Input: part model. Units: mm. Frame: model coordinates. Round coordinates to 2 decimals unless told otherwise and drop trailing zeros. Order: outer loops, then holes, each group sorted by start corner. A loop starts at its lowest first (then second) coordinate and runs counter-clockwise, first axis right, second up. Notation, with made-up numbers: (-13, 12) -> (35, 12) arc R20 cw to (35, 43) -> close; hole circle Ø11 at (43.5, 20.25). An arc over 180 degrees is marked (long way). Answer as CSV lines item,"result". Start each with the question number.
1) Section query D-D, the plane z = 19. Output: boundary loops of the cut face in (x, y) (3 decimals).
2) Line query: L1, parallel to Z at x = -3.4, y = 142.24; L2, parallel to Z at x = -5.5, y = 130 (3 decimals); L3, parallel to X at y = 31, z = 76. Output: solid intervals per line, ascending.
3) Section query C-C, the plane y = 78. Output: boundary loops of the cut face in (x, z) (3 decimals), and give its area (3 significant figures).
4) Section query A-A, the plane z = 78.5. Output: boundary loops of the cut face in (x, y).
5) First-contact query: P1, Ø7.5, axis at y = 24.18, z = -24.05, coming from the -X side; P2, Ø3, axis at x = -9, y = 117.5, coming from the -Z side; P3, Ø10, axis at x = -18.5, y = -3, coming from the +Z side (3 decimals); P4, Ø4, axis at y = 19.5, z = -23, coming from the +X side. Flat tips, straight axial feed; report the tip coordinate or a pass-through.
6) Section query B-B, the plane x = -28. Output: boundary loops of the cut face in (y, z) (3 decimals), and give its area (3 significant figures).
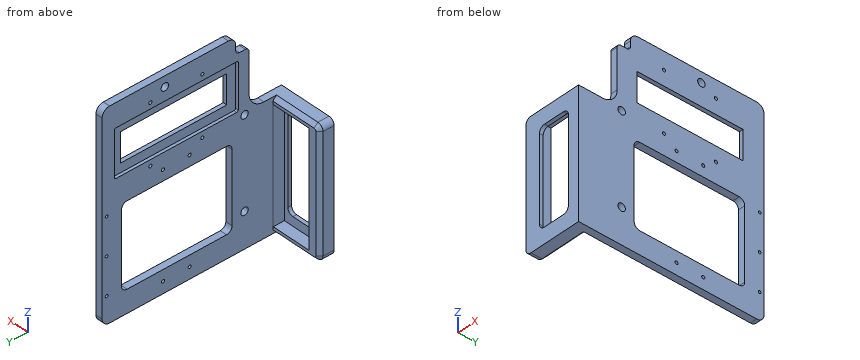
Autodesk Inventor part; units mm, degrees
ref_plane "YZ Plane" through (0, 0, 0) normal (1, 0, 0) x (0, 1, 0)
ref_plane "XZ Plane" through (0, 0, 0) normal (0, 1, 0) x (-1, 0, 0)
ref_plane "XY Plane" through (0, 0, 0) normal (0, 0, 1) x (1, 0, 0)
sketch "Sketch1" plane through (0, 0, 0) normal (0, 1, 0) x (-1, 0, 0)
  line L0 (0, -75.565) -> (0, 75.565)
  line L1 (-9.8806, 0) -> (59.2836, 0)
  line L2 (36.703, -40.64) -> (9.525, -40.64)
  line L3 (9.525, -40.64) -> (9.525, 40.64)
  line L4 (9.525, 40.64) -> (36.703, 40.64)
  line L5 (36.703, 40.64) -> (36.703, -40.64)
  line L6 (36.703, -40.64) -> (9.525, 40.64) construction
  line L7 (9.525, -40.64) -> (36.703, 40.64) construction
  line L8 (0, -53.975) -> (49.403, -53.975)
  line L9 (49.403, -53.975) -> (49.403, 53.975)
  line L10 (49.403, 53.975) -> (0, 53.975)
  line L11 (0, 53.975) -> (0, -53.975)
  line L12 (0, -53.975) -> (49.403, 53.975) construction
  line L13 (49.403, -53.975) -> (0, 53.975) construction
  point P0 (0, 0)
  point P1 (23.114, 0)
  point P2 (24.7015, 0)
  dimension "d0" = 81.28
  dimension "d1" = 27.178
  dimension "d3" = 107.95
  dimension "d4" = 12.7
  dimension "d6" = 9.525
  dimension "d7" = 0
extrude "Extrusion1" add sketch "Sketch1" against normal blind 12.7 contours L0 L1 L3 L2 L5 L9 L8 | L0 L10 L9 L1 L5 L4 L3
sketch "Sketch2" plane through (0, 0, 0) normal (0, 1, 0) x (1, 0, 0)
  point P0 (0, 0)
sketch "Sketch4" plane through (0, 0, 0) normal (0, 1, 0) x (1, 0, 0)
  point P0 (0, 0)
sketch "Sketch5" plane through (0, 0, 0) normal (0, 1, 0) x (1, 0, 0)
  line L0 (9.8806, 0) -> (-59.2836, 0)
  line L1 (0, 75.565) -> (0, -75.565)
  line L2 (-39.878, 48.26) -> (-6.223, 48.26)
  line L3 (-6.223, 48.26) -> (-6.223, -48.26)
  line L4 (-6.223, -48.26) -> (-39.878, -48.26)
  line L5 (-39.878, -48.26) -> (-39.878, 48.26)
  line L6 (-39.878, 48.26) -> (-6.223, -48.26) construction
  line L7 (-6.223, 48.26) -> (-39.878, -48.26) construction
  line L8 (-9.525, 40.64) -> (-9.525, -40.64)
  point P0 (0, 0)
  point P1 (-23.0505, 0)
  dimension "d13" = 3.302
  dimension "d14" = 96.52
  dimension "d15" = 33.655
extrude "Extrusion3" cut sketch "Sketch5" against normal blind 9.525
sketch "Sketch3" plane through (0, 0, 53.975) normal (1, 0, 0) x (0, 0, -1)
  line L0 (0, 0) -> (0, -12.7)
  line L1 (0, 0) -> (107.95, 0)
  line L2 (107.95, 0) -> (107.95, -12.7)
  line L3 (107.95, 146.05) -> (0, 146.05)
  line L4 (0, 146.05) -> (0, 0)
  line L5 (0, 0) -> (107.95, 0)
  line L6 (107.95, 0) -> (107.95, 146.05)
  line L7 (107.95, 146.05) -> (0, 0) construction
  line L8 (0, 146.05) -> (107.95, 0) construction
  line L9 (0, 20.32) -> (-63.5, 20.32)
  line L10 (-63.5, 20.32) -> (-63.5, 146.05)
  line L11 (-63.5, 146.05) -> (0, 146.05)
  line L12 (107.95, -12.7) -> (0, -12.7)
  line L13 (-49.53, 20.32) -> (-49.53, 31.75)
  line L14 (-49.53, 31.75) -> (-63.5, 31.75)
  point P0 (53.975, 0)
  point P1 (53.975, 73.025)
  point P2 (1.8288, 24.1808)
  point P3 (78.0288, 24.1808)
  point P4 (-54.7116, 92.3798)
  dimension "d10" = 146.05
  dimension "d18" = 33.02
  dimension "d19" = 63.5
  dimension "d20" = 13.97
  dimension "d21" = 11.43
  dimension "d22" = 36.8808
  dimension "d23" = 29.9212
  dimension "d24" = 106.1212
  dimension "d32" = 162.6616
  dimension "d33" = 105.0798
extrude "Extrusion2" add sketch "Sketch3" against normal blind 5.842 contours L4 L3 L6 L1 | L9 L13 L14 L10 L11 L4
hole "Hole1" at (0, 24.1808, -24.0538) at (0, 24.1808, 52.1462) at (0, 92.3798, 108.6866) direction (-1, 0, 0) diameter 6.35 end through all
sketch "Sketch6" plane through (-5.842, 0, 53.975) normal (-1, 0, 0) x (0, 0, 1)
  line L0 (3.495, 135.55) -> (43.495, 135.55)
  line L1 (43.495, 135.55) -> (43.495, 29.55)
  line L2 (43.495, 29.55) -> (3.495, 29.55)
  line L3 (3.495, 29.55) -> (3.495, 135.55)
  line L4 (3.495, 135.55) -> (43.495, 29.55) construction
  line L5 (43.495, 135.55) -> (3.495, 29.55) construction
  line L6 (0, -12.7) -> (-107.95, -12.7)
  line L7 (-107.95, 0) -> (-107.95, -12.7)
  line L8 (48.575, 104.775) -> (-1.585, 104.775) construction
  line L9 (-1.585, 104.775) -> (-1.585, 60.325) construction
  line L10 (-1.585, 60.325) -> (48.575, 60.325) construction
  line L11 (48.575, 60.325) -> (48.575, 104.775) construction
  line L12 (48.575, 104.775) -> (-1.585, 60.325) construction
  line L13 (-1.585, 104.775) -> (48.575, 60.325) construction
  line L14 (-53.975, 177.8) -> (-53.975, -44.45) construction
  line L15 (-142.24, 0) -> (97.79, 0) construction
  line L16 (-98.1075, 93.98) -> (-9.8425, 93.98) construction
  line L17 (-9.8425, 93.98) -> (-9.8425, 71.12) construction
  line L18 (-9.8425, 71.12) -> (-98.1075, 71.12) construction
  line L19 (-98.1075, 71.12) -> (-98.1075, 93.98) construction
  line L20 (-98.1075, 93.98) -> (-9.8425, 71.12) construction
  line L21 (-9.8425, 93.98) -> (-98.1075, 71.12) construction
  point P0 (-53.975, 0)
  point P1 (23.495, 82.55)
  point P2 (-53.975, 82.55)
  dimension "d36" = 40
  dimension "d37" = 106
  dimension "d38" = 95.25
  dimension "d39" = 131.445
  dimension "d43" = 5.08
  dimension "d44" = 44.45
  dimension "d45" = 88.265
  dimension "d46" = 22.86
  dimension "d47" = 106.68
extrude "Extrusion4" cut sketch "Sketch6" against normal blind 2.54
fillet "Fillet3" radius 1.27 4 edges at (-4.572, 29.55, 97.47) (-4.572, 29.55, 57.47) (-4.572, 135.55, 57.47) (-4.572, 135.55, 97.47)
hole "Hole2" at (-5.842, 93.98, 44.1325) at (-5.842, 71.12, 44.1325) at (-5.842, 71.12, -44.1325) at (-5.842, 93.98, -44.1325) at (-5.842, 104.775, 52.39) at (-5.842, 60.325, 52.39) at (-5.842, 60.325, 102.55) at (-5.842, 104.775, 102.55) direction (1, 0, 0) diameter 2.6416 end through all
fillet "Fillet1" radius 3.175 2 edges at (-2.921, 31.75, 103.505) (-2.921, 20.32, 103.505)
fillet "Fillet2" radius 12.7 1 edges at (-2.921, 20.32, 53.975)
sketch "Sketch7" plane through (-5.842, 0, 53.975) normal (-1, 0, 0) x (0, 0, 1)
  line L0 (-98.1075, 93.98) -> (-9.8425, 93.98) construction
  circle A0 centre (-9.8425, 93.98) radius 1.3208 construction
  line L1 (-98.1075, 142.24) -> (-9.8425, 142.24) construction
  line L2 (-9.8425, 142.24) -> (-9.8425, 93.98) construction
  line L3 (-9.8425, 93.98) -> (-98.1075, 93.98) construction
  line L4 (-98.1075, 93.98) -> (-98.1075, 142.24) construction
  line L5 (-98.1075, 142.24) -> (-9.8425, 93.98) construction
  line L6 (-9.8425, 142.24) -> (-98.1075, 93.98) construction
  line L7 (63.5, 146.05) -> (-107.95, 146.05) construction
  point P0 (-53.975, 0)
  point P1 (-53.975, 118.11)
  point P2 (-53.975, 142.24)
  point P3 (-22.5425, 142.24)
  point P4 (-85.4075, 142.24)
  dimension "d55" = 3.81
  dimension "d75" = 12.7
  dimension "d76" = 12.7
hole "Hole3" at (-5.842, 142.24, 0) at (-5.842, 142.24, 31.4325) at (-5.842, 142.24, -31.4325) direction (1, 0, 0) diameter 2.3622 end through all
fillet "Fillet4" radius 6.35 3 edges at (-2.921, 146.05, 117.475) (-2.921, 146.05, -53.975) (-2.921, 31.75, 117.475)
fillet "Fillet5" radius 4.7625 2 edges at (-49.403, -6.35, 53.975) (-49.403, -6.35, -53.975)
sketch "Sketch8" plane through (-5.842, 0, 53.975) normal (-1, 0, 0) x (0, 0, 1)
  line L0 (-88.7872, 129.4659) -> (-18.9372, 129.4659)
  line L1 (-18.9372, 129.4659) -> (-18.9372, 34.8509)
  line L2 (-18.9372, 34.8509) -> (-88.7872, 34.8509)
  line L3 (-88.7872, 34.8509) -> (-88.7872, 129.4659)
  line L4 (-88.7872, 129.4659) -> (-18.9372, 34.8509) construction
  line L5 (-18.9372, 129.4659) -> (-88.7872, 34.8509) construction
  point P0 (-53.975, 0)
  point P1 (-53.8622, 82.1584)
  dimension "d65" = 69.85
  dimension "d66" = 94.615
extrude "Extrusion5" cut sketch "Sketch8" against normal through all
fillet "Fillet6" radius 4.7625 4 edges at (-2.921, 129.4659, 35.0378) (-2.921, 34.8509, -34.8122) (-2.921, 129.4659, -34.8122) (-2.921, 34.8509, 35.0378)
sketch "Sketch9" plane through (-3.302, 0, 53.975) normal (-1, 0, 0) x (0, 0, 1)
  arc A0 (43.495, 134.28) -> (42.225, 135.55) centre (42.225, 134.28) ccw
  line L0 (4.765, 135.55) -> (42.225, 135.55)
  arc A1 (4.765, 135.55) -> (3.495, 134.28) centre (4.765, 134.28) ccw
  line L1 (3.495, 30.82) -> (3.495, 134.28)
  arc A2 (3.495, 30.82) -> (4.765, 29.55) centre (4.765, 30.82) ccw
  line L2 (42.225, 29.55) -> (4.765, 29.55)
  arc A3 (42.225, 29.55) -> (43.495, 30.82) centre (42.225, 30.82) ccw
  line L3 (43.495, 134.28) -> (43.495, 30.82)
  line L4 (11.0923, 37.1473) -> (11.0923, 127.9527)
  line L5 (11.0923, 127.9527) -> (35.8977, 127.9527)
  line L6 (35.8977, 127.9527) -> (35.8977, 37.1473)
  line L7 (35.8977, 37.1473) -> (11.0923, 37.1473)
  point P0 (-53.975, 0)
  point P1 (23.495, 82.55)
extrude "Extrusion6" cut sketch "Sketch9" against normal through all contours L4 L5 L6 L7
chamfer "Chamfer1" distance 3.175 angle 45 5 edges at (-25.2413, 0, -53.975) (-48.0081, 0, -52.5801) (-49.403, 0, 0) (-48.0081, 0, 52.5801) (-25.2412, 0, 53.975)
fillet "Fillet7" radius 4.7625 4 edges at (-36.703, -11.1125, 40.64) (-9.525, -11.1125, 40.64) (-9.525, -11.1125, -40.64) (-36.703, -11.1125, -40.64)
properties material "ABS, BLACK"
Findings:
1,outline,"(-49.403, -12.7) -> (-36.703, -12.7) -> (-36.703, -9.525) -> (-39.878, -9.525) -> (-39.878, 0) -> (-46.228, 0) -> (-49.403, -3.175) -> close; (-9.525, -12.7) -> (0, -12.7) -> (0, 34.851) -> (-5.842, 34.851) -> (-5.842, 0) -> (-6.223, 0) -> (-6.223, -9.525) -> (-9.525, -9.525) -> close; (-5.842, 129.466) -> (0, 129.466) -> (0, 146.05) -> (-5.842, 146.05) -> close"
2,L1,"z = -53.44 to -32.61, -30.25 to -1.18, 1.18 to 30.25, 32.61 to 116.94"
2,L2,"z = -53.975 to 57.47, 97.47 to 117.475"
2,L3,"x = -3.3 to 0"
3,outline,"(-5.842, -53.975) -> (0, -53.975) -> (0, -34.812) -> (-5.842, -34.812) -> close; (-5.842, 35.038) -> (0, 35.038) -> (0, 65.067) -> (-3.302, 65.067) -> (-3.302, 57.47) -> (-5.842, 57.47) -> close; (-5.842, 97.47) -> (-3.302, 97.47) -> (-3.302, 89.873) -> (0, 89.873) -> (0, 117.475) -> (-5.842, 117.475) -> close"
3,area,"410 mm^2"
4,outline,"(-5.84, 20.32) -> (0, 20.32) -> (0, 37.15) -> (-3.3, 37.15) -> (-3.3, 29.55) -> (-5.84, 29.55) -> close; (-5.84, 135.55) -> (-3.3, 135.55) -> (-3.3, 127.95) -> (0, 127.95) -> (0, 146.05) -> (-5.84, 146.05) -> close"
5,P1,"stops at x = -5.84"
5,P2,"passes through"
5,P3,"stops at z = 53.975"
5,P4,"stops at x = 0"
6,outline,"(-12.7, -53.975) -> (-3.175, -53.975) -> (0, -50.8) -> (0, -48.26) -> (-9.525, -48.26) -> (-9.525, -40.64) -> (-12.7, -40.64) -> close; (-12.7, 40.64) -> (-9.525, 40.64) -> (-9.525, 48.26) -> (0, 48.26) -> (0, 50.8) -> (-3.175, 53.975) -> (-12.7, 53.975) -> close"
6,area,"183 mm^2"
